from build123d import *

# Parameters (mm, degrees)
BOSS_EXTRU_1_DEPTH      = 11
BOSS_EXTRU_2_DEPTH      = 26
BOSS_EXTRU_3_DEPTH      = 11
ESQUISSE4_R             = 11
BOSS_EXTRU_4_DEPTH      = 2
ESQUISSE5_R             = 2.5
BOSS_EXTRU_5_DEPTH      = 20
ESQUISSE6_W             = 5.798316384
ESQUISSE6_H             = 1
ENL_V_MAT_EXTRU_1_DEPTH = 18
TROU_TARAUD_M31_D       = 2.5
TROU_TARAUD_M31_DEPTH   = 7
TROU_TARAUD_M31_TIP     = 0.751075774
ESQUISSE9_W             = 6.3
ESQUISSE9_H             = 4.75
BOSS_EXTRU_6_DEPTH      = 2.3
ESQUISSE10_R            = 0.2025
BOSS_EXTRU_7_DEPTH      = 10
ESQUISSE11_R            = 0.55
BOSS_EXTRU_8_DEPTH      = 8


with BuildPart() as part:
    # Esquisse1 → Boss.-Extru.1 (new body)
    with BuildSketch(Plane.XY):
        Polygon((17, 21), (21, 17), (21, -17), (17, -21), (-17, -21), (-21, -17), (-21, 17), (-17, 21), align=None)
    extrude(amount=BOSS_EXTRU_1_DEPTH)

    # Esquisse2 → Boss.-Extru.2 (add)
    with BuildSketch(Plane(origin=(0, 0, 0), x_dir=(-1, 0, 0), z_dir=(0, 0, -1))):
        Polygon((-16, 21), (16, 21), (21, 16), (21, -16), (16, -21), (-16, -21), (-21, -16), (-21, 16), align=None)
    extrude(amount=BOSS_EXTRU_2_DEPTH)

    # Esquisse3 → Boss.-Extru.3 (add)
    with BuildSketch(Plane(origin=(0, 0, -26), x_dir=(-1, 0, 0), z_dir=(0, 0, -1))):
        Polygon((-17, 21), (-21, 17), (-21, -17), (-17, -21), (17, -21), (21, -17), (21, 17), (17, 21), align=None)
    extrude(amount=BOSS_EXTRU_3_DEPTH)

    # Esquisse4 → Boss.-Extru.4 (add)
    with BuildSketch(Plane(origin=(0, 0, -37), x_dir=(-1, 0, 0), z_dir=(0, 0, -1))):
        Circle(ESQUISSE4_R)
    extrude(amount=BOSS_EXTRU_4_DEPTH)

    # Esquisse5 → Boss.-Extru.5 (add)
    with BuildSketch(Plane(origin=(0, 0, -39), x_dir=(-1, 0, 0), z_dir=(0, 0, -1))):
        Circle(ESQUISSE5_R)
    extrude(amount=BOSS_EXTRU_5_DEPTH)

    # Esquisse6 → Enlèv. mat.-Extru.1 (cut)
    with BuildSketch(Plane(origin=(0, 0, -59), x_dir=(-1, 0, 0), z_dir=(0, 0, -1))):
        with Locations((0, 2.5)):
            Rectangle(ESQUISSE6_W, ESQUISSE6_H)
    extrude(amount=-ENL_V_MAT_EXTRU_1_DEPTH, mode=Mode.SUBTRACT)

    # Trou taraudé M31
    with Locations(Plane(origin=(0, 0, -37), x_dir=(-1, 0, 0), z_dir=(0, 0, -1))):
        with Locations((-15.5, 15.5), (15.5, 15.5), (15.5, -15.5), (-15.5, -15.5)):
            Hole(TROU_TARAUD_M31_D / 2, depth=TROU_TARAUD_M31_DEPTH)
            with Locations((0, 0, -(TROU_TARAUD_M31_DEPTH + TROU_TARAUD_M31_TIP / 2))):  # 118° drill point
                Cone(0, TROU_TARAUD_M31_D / 2, TROU_TARAUD_M31_TIP, mode=Mode.SUBTRACT)

    # Esquisse9 → Boss.-Extru.6 (add)
    with BuildSketch(Plane.XZ.offset(21)):
        with Locations((0, 6.925)):
            Rectangle(ESQUISSE9_W, ESQUISSE9_H)
    extrude(amount=BOSS_EXTRU_6_DEPTH)

    # Esquisse10 → Boss.-Extru.7 (add)
    with BuildSketch(Plane.XZ.offset(23.3)):
        with Locations(Location((-2.25, 6.925, 0), (0, 0, 270))):
            Circle(ESQUISSE10_R)
        with Locations(Location((-0.75, 6.925, 0), (0, 0, 270))):
            Circle(ESQUISSE10_R)
        with Locations(Location((0.75, 6.925, 0), (0, 0, 270))):
            Circle(ESQUISSE10_R)
        with Locations(Location((2.25, 6.925, 0), (0, 0, 270))):
            Circle(ESQUISSE10_R)
    extrude(amount=BOSS_EXTRU_7_DEPTH)

    # Esquisse11 → Boss.-Extru.8 (add)
    with BuildSketch(Plane.XZ.offset(23.3)):
        with Locations(Location((-2.25, 6.925, 0), (0, 0, 270))):
            Circle(ESQUISSE11_R)
        with Locations(Location((-0.75, 6.925, 0), (0, 0, 270))):
            Circle(ESQUISSE11_R)
        with Locations(Location((0.75, 6.925, 0), (0, 0, 270))):
            Circle(ESQUISSE11_R)
        with Locations(Location((2.25, 6.925, 0), (0, 0, 270))):
            Circle(ESQUISSE11_R)
    extrude(amount=BOSS_EXTRU_8_DEPTH)


solid = part.part
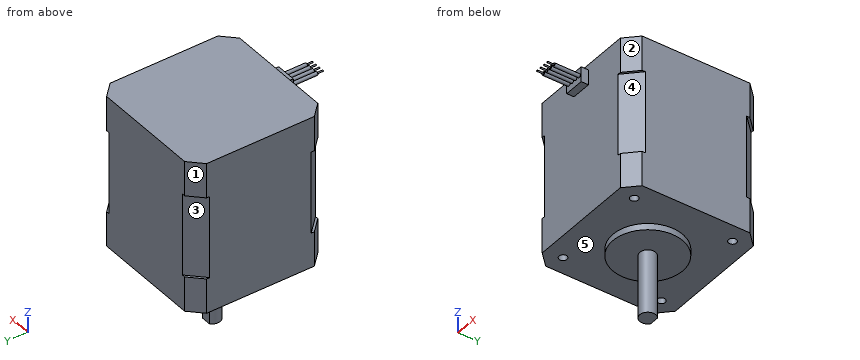
Input: part model. Units: mm. Frame: model coordinates. Face numbers are marked on the shaded views. A direction names the side the tool comes from. Give positions to 0.01 mm unless a question says otherwise; leave off trailing zeros. Order: outer loops, then holes, each group sorted by start corner. A loop starts at its lowest first (then second) coordinate and runs counter-clockwise, first axis right, second up. Notation, with made-up numbers: (28.25, 47) - (46.25, 47) arc R21 ccw to (46.25, 68) - close; hole circle Ø5 at (39, 53.25). An arc over 180 degrees is marked (long way). Answer as a JSON object with one key per item and string values. Group by question number.
Q1. Cut plane B-B, the plane y = 0. Output: boundary loops of the cut face in (x, z).
Q2. Cut plane C-C, the plane z = -33.5. Output: boundary loops of the cut face in (x, y), then the cut area to 3 significant figures.
Q3. Line query: probe 1 along Y at (x, z) = (-15.5, -33); probe 2 along Y at (x, z) = (-15, -33). Output: solid intervals per line, ascending.
Q4. Cut plane D-D, the plane x = -10. Output: boundary loops of the cut face in (y, z).
Q5. Set-up query: the marked faces 1, 2, 3, 4 and 5. Return all of +Z, -Z, +X, -X, +Y, -Y with unobstructed straight access to the full face (end or side cutting, diameter ignored); none if empty.
Q6. First-contact query: pin 1 Ø10 at (x, z) = (-7, -9) entering from -Y; pin 2 Ø5.5 at (x, y) = (-17.5, 18.5) entering from -Z; pin 3 Ø0.6 at (x, y) = (0.5, 2.5) entering from -Z. Flat tips, straight axial feed; report the tip coordinate or a pass-through.
Q7. Cut plane A-A, the plane z = -17.5. Output: boundary loops of the cut face in (x, y), then the cut area to 3 significant figures.
Results:
{
 "1": {"outline": "(-21, -37) - (-11, -37) - (-11, -39) - (-2.5, -39) - (-2.5, -59) - (2.5, -59) - (2.5, -39) - (11, -39) - (11, -37) - (21, -37) - (21, 11) - (-21, 11) - close"},
 "2": {"outline": "(-21, -17) - (-17, -21) - (17, -21) - (21, -17) - (21, 17) - (17, 21) - (-17, 21) - (-21, 17) - close; hole circle Ø2.5 at (-15.5, -15.5); hole circle Ø2.5 at (-15.5, 15.5); hole circle Ø2.5 at (15.5, -15.5); hole circle Ø2.5 at (15.5, 15.5)", "area": "1,710 mm^2"},
 "3": {"probe 1": "-21 to -16.75, -14.25 to 14.25, 16.75 to 21", "probe 2": "-21 to -16.65, -14.35 to 14.35, 16.65 to 21"},
 "4": {"outline": "(-21, -37) - (-4.58, -37) - (-4.58, -39) - (4.58, -39) - (4.58, -37) - (21, -37) - (21, 11) - (-21, 11) - close"},
 "5": {"face 1": "+Z, -Z, -X, +Y", "face 2": "+Z, -Z, +X, -Y", "face 3": "-X, +Y", "face 4": "+X, -Y", "face 5": "-Z"},
 "6": {"pin 1": "y = -21", "pin 2": "z = -37", "pin 3": "z = -41"},
 "7": {"outline": "(-21, -16) - (-16, -21) - (16, -21) - (21, -16) - (21, 16) - (16, 21) - (-16, 21) - (-21, 16) - close", "area": "1,710 mm^2"}
}
